Geometry: final body of the model. Coordinates: model frame, mm. Face numbers are marked on the shaded views. A direction names the side the tool comes from. Give positions to 0.01 mm unless a question says otherwise; leave off trailing zeros. Write each loop counter-clockwise with the first axis right and the second up, starting at its lowest first coordinate (ties: lowest second). Pieces come first, ordered by that corner, then holes. Notation, with made-up numbers: M 82.25,2.25 L 105.25,2.25 A25 ccw 105.25,35.25 Z; hole C -35.5,52 d3. An arc over 180 degrees is marked long. Use a Markdown table: item, result. Add a question column.
1) Section A-A on x = 0. State how many separate pieces and enclosed holes the cut face has, then the cut area to 3 significant figures.
2) Line query: line 1 (X direction, y = 0, z = -10.5) (3 decimals); line 2 (Z direction, x = 23, y = 21); line 3 (Y direction, x = 7.5, z = -9.5). Output: solid intervals per line, ascending.
3) Set-up query: the marked faces 1 and 2. Return all of +Z, -Z, +X, -X, +Y, -Y with unobstructed straight access to the full face (end or side cutting, diameter ignored); none if empty.
4) Draft query along Y for the marked faces 3, 4 and 5. Return one class per face: +Y half, -Y half, draft (parallel to the pull), parting line (faces both ways), or undercut.
5) Section C-C on z = -30.5. Return the cut outline in (x, y) (3 decimals), then the cut area to 3 significant figures.
6) Section D-D on x = 38.5. Return the cut outline in (y, z), then the cut area to 3 significant figures.
7) Pin query (flat end, axial travel): pin 1 (14.5 mm diameter, centred on x = 0, y = -39.69, fed in from +Z); pin 2 (10 mm diameter, centred on y = 19, z = -39.5, fed in from -X); pin 3 (1 mm diameter, centred on x = 4, z = -27.5, fed in from -Y); pin 4 (3 mm diameter, centred on x = 6, z = -16.5, fed in from -Y). Return the tip coordinate at first contact, or that it passes through.
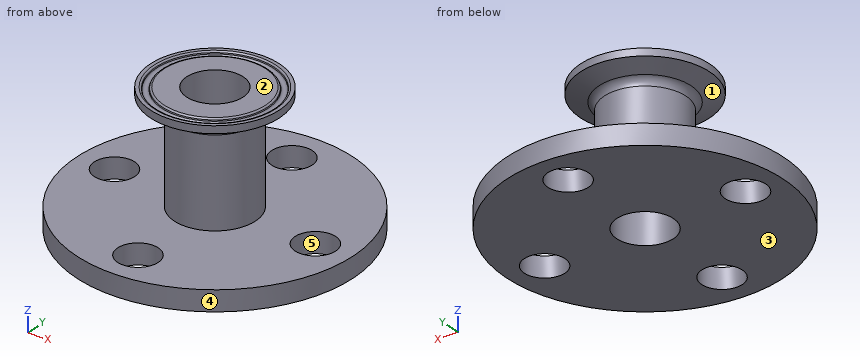
```python
from build123d import *

# Parameters (mm, degrees)
SKETCH2_R          = 7.9375
CUT_EXTRUDE1_DEPTH = 7.9375


with BuildPart() as part:
    # Sketch1 → Revolve1 (revolve)
    with BuildSketch(Plane(origin=(0, 0, 0), x_dir=(0, 0, -1), z_dir=(1, 0, 0))):
        with BuildLine():
            Line((0, 11.049), (0, 19.828027725))
            ThreePointArc((0, 19.828027725), (0.130798304, 20.262622907), (0.479738309, 20.552833247))
            Line((0.479738309, 20.552833247), (0.872854821, 20.719701306))
            ThreePointArc((0.872854821, 20.719701306), (1.6002, 21.8186), (0.872854821, 22.917498694))
            Line((0.872854821, 22.917498694), (0.479738309, 23.084366753))
            ThreePointArc((0.479738309, 23.084366753), (0.130798304, 23.374577093), (0, 23.809172275))
            Line((0, 23.809172275), (0, 25.1968))
            Line((0, 25.1968), (2.8448, 25.1968))
            Line((2.8448, 25.1968), (5.477292593, 17.964086045))
            ThreePointArc((5.477292593, 17.964086045), (6.639711478, 16.449192259), (8.460816664, 15.875))
            Line((8.460816664, 15.875), (42.8625, 15.875))
            Line((42.8625, 15.875), (42.8625, 53.975))
            Line((42.8625, 53.975), (50.8, 53.975))
            Line((50.8, 53.975), (50.8, 28.575))
            Line((50.8, 28.575), (50.8, 11.049))
            Line((50.8, 11.049), (0, 11.049))
        make_face()
    revolve(axis=Axis((0, 0, 0), (0, 0, -1)))

    # Sketch2 → Cut-Extrude1 (cut)
    with BuildSketch(Plane(origin=(0, 0, -50.8), x_dir=(-1, 0, 0), z_dir=(0, 0, -1))):
        with Locations((0, 39.6875)):
            Circle(SKETCH2_R)
        with Locations((39.6875, 0)):
            Circle(SKETCH2_R)
        with Locations((0, -39.6875)):
            Circle(SKETCH2_R)
        with Locations((-39.6875, 0)):
            Circle(SKETCH2_R)
    extrude(amount=-CUT_EXTRUDE1_DEPTH, mode=Mode.SUBTRACT)


solid = part.part
```
Found:
| question | item | result |
|---|---|---|
| 1 | separate pieces | 4 |
| 1 | enclosed holes | 0 |
| 1 | area | 923 mm² |
| 2 | line 1 | -15.875 to -11.049, 11.049 to 15.875 |
| 2 | line 2 | -50.8 to -42.86 |
| 2 | line 3 | -13.99 to -8.11, 8.11 to 13.99 |
| 3 | face 1 | none |
| 3 | face 2 | +Z, +X, -X, +Y, -Y |
| 4 | face 3 | draft |
| 4 | face 4 | parting line |
| 4 | face 5 | undercut |
| 5 | outline | C 0,0 d31.75; hole C 0,0 d22.098 |
| 5 | area | 408 mm² |
| 6 | outline | M -37.83,-50.8 L -7.85,-50.8 L -7.85,-42.86 L -37.83,-42.86 Z; M 7.85,-50.8 L 37.83,-50.8 L 37.83,-42.86 L 7.85,-42.86 Z |
| 6 | area | 476 mm² |
| 7 | pin 1 | through |
| 7 | pin 2 | x = -51.76 |
| 7 | pin 3 | y = -15.48 |
| 7 | pin 4 | y = -15.22 |
